Build history of the part. All positions in model axes, mm. A direction names the side the tool comes from. Coordinates: 2 decimals unless noted, no trailing zeros. Write each loop counter-clockwise with the first axis right and the second up, starting at its lowest first coordinate (ties: lowest second). Pieces come first, ordered by that corner, then holes.
from build123d import *

# Parameters (mm, degrees)
F0_W     = 20
F0_H     = 10
F0_W_2   = 5
F0_H_2   = 3
F1_DEPTH = 3
F2_R     = 4.99999
F4_D     = 3


# Not quite as in the source:
# - a fillet or chamfer is up to 0.001 mm smaller than in the source, because OpenCascade refuses the exact size


with BuildPart() as f1:
    # F0 (on Top) → F1 (new body)
    with BuildSketch(Plane.XY):
        Rectangle(F0_W, F0_H)
        Rectangle(F0_W_2, F0_H_2, mode=Mode.SUBTRACT)
    extrude(amount=-F1_DEPTH)

    # F2 (radius 5 in the source; OpenCascade refuses exactly that, so slightly less here)
    f2_edges = [f1.edges().sort_by_distance(p)[0] for p in [
        (-10, -5, -1.5),
        (-10, 5, -1.5),
        (10, -5, -1.5),
        (10, 5, -1.5),
    ]]
    fillet(f2_edges, radius=F2_R)

    # F4 (through all)
    with Locations(Plane.XY):
        with Locations((-7, 0), (7, 0)):
            Hole(F4_D / 2)


solid = f1.part
(1) Probe L1, parallel to X at y = -0.5, z = -2.55; L2, parallel to X at y = -1.25, z = -2.7; L3, parallel to Y at x = 1, z = -1.2. List the from-to ranges inside material, lowest first.
(2) Slice it at D-D, the plane x = 8. List the corners of the cut face in (y, z).
(3) Two-plate mould, pull along X, no slides. Class faces 3 (the cylindrical face through (-5.5, 0.07, -1.52)), 4 (the flat face through (0, -2, 0)), 5 (the cylindrical face through (8, 4, -2)), 6 (the cylindrical face through (-9, 3, -2)): pulls with the +X half, pulls with the -X half, needs draft (parallel to the pull), parting line crosses it, or undercut.
(4) Slice it at C-C, the plane y = -0.75. List the corners of the cut face in (x, z), and give its area (3 significant figures).
(5) Slice it at A-A, the plane x = 1.5. List the corners of the cut face in (y, z), and give its area (3 significant figures).
(6) Flat gauge pin, fed straight in: P1, Ø2.5, axis at x = -7, y = 0, coming from the -Z side. Where does the tip first touch, or does it go through?
(7) 3-axis set-ups, long thin cutter, end or side, ignore diameter. For faces 1 (the flat face through (0, -2, -3)), 2 (the flat face through (0, -1.5, -1)): which of +Z, -Z, +X, -X, +Y, -Y reach the whole face in a straight line?
(8) Slice it at B-B, the plane z = -0.9. Give the number of separate pieces and of enclosed holes in the cut face, and give its area (3 significant figures).
Results:
1. L1: x = -9.97 to -8.41, -5.59 to -2.5, 2.5 to 5.59, 8.41 to 9.97
1. L2: x = -9.84 to -7.83, -6.17 to -2.5, 2.5 to 6.17, 7.83 to 9.84
1. L3: y = -5 to -1.5, 1.5 to 5
2. outline: (-4, -3) - (-1.12, -3) - (-1.12, 0) - (-4, 0) - close; (1.12, -3) - (4, -3) - (4, 0) - (1.12, 0) - close
3. face 3: undercut
3. face 4: needs draft
3. face 5: pulls with the +X half
3. face 6: pulls with the -X half
4. outline: (-9.94, -3) - (-8.3, -3) - (-8.3, 0) - (-9.94, 0) - close; (-5.7, -3) - (-2.5, -3) - (-2.5, 0) - (-5.7, 0) - close; (2.5, -3) - (5.7, -3) - (5.7, 0) - (2.5, 0) - close; (8.3, -3) - (9.94, -3) - (9.94, 0) - (8.3, 0) - close
4. area: 29.1 mm2
5. outline: (-5, -3) - (-1.5, -3) - (-1.5, 0) - (-5, 0) - close; (1.5, -3) - (5, -3) - (5, 0) - (1.5, 0) - close
5. area: 21.0 mm2
6. P1: passes through
7. face 1: -Z, +X, -X, +Y, -Y
7. face 2: +Z, -Z
8. separate pieces: 1
8. enclosed holes: 3
8. area: 149 mm2
